```python
from build123d import *

# Parameters (mm, degrees)
RESSALTO_EXTRUS_O1_DEPTH = 50
ESBO_O2_R                = 4
CORTE_EXTRUS_O1_DEPTH    = 24
CORTE_EXTRUS_O2_DEPTH    = 51
FILETE1_R                = 10


with BuildPart() as part:
    # Esboço1 → Ressalto-extrusão1 (new body)
    with BuildSketch(Plane.XY):
        Polygon((87.5, 0), (-87.5, 0), (-87.5, 23), (-20, 23), (-20, 85), (20, 85), (20, 23), (87.5, 23), align=None)
    extrude(amount=RESSALTO_EXTRUS_O1_DEPTH)

    # Esboço2 → Corte-extrusão1 (cut, through all)
    with BuildSketch(Plane(origin=(0, 23, 0), x_dir=(1, 0, 0), z_dir=(0, 1, 0))):
        with Locations((-67.5, -25)):
            Circle(ESBO_O2_R)
        with Locations((67.5, -25)):
            Circle(ESBO_O2_R)
    extrude(amount=-CORTE_EXTRUS_O1_DEPTH, mode=Mode.SUBTRACT)

    # Esboço3 → Corte-extrusão2 (cut, through all)
    with BuildSketch(Plane.XY.offset(50)):
        with BuildLine():
            Line((1, 62.660568708), (1, 116.5))
            Line((1, 116.5), (-1, 116.5))
            Line((-1, 116.5), (-1, 62.660568708))
            ThreePointArc((-1, 62.660568708), (0, 37.3), (1, 62.660568708))
        make_face()
    extrude(amount=-CORTE_EXTRUS_O2_DEPTH, mode=Mode.SUBTRACT)

    # Filete1
    filete1_edges = [part.edges().sort_by_distance(p)[0] for p in [
        (-20, 23, 25),
        (20, 23, 25),
    ]]
    fillet(filete1_edges, radius=FILETE1_R)

    # Esboço5 → Rebaixo para parafuso de máquina com cabeça panela de M61 (revolve, cut)
    with BuildSketch(Plane(origin=(20, 74.5, 25), x_dir=(0, 0, -1), z_dir=(0, 1, 0))):
        Polygon((0, 0), (0, 107.5), (3.3, 107.5), (3.3, 4.6), (6.5, 4.6), (6.5, 0.025), (6.525, 0), align=None)
    revolve(axis=Axis((26.35, 74.5, 25), (-1, 0, 0)), mode=Mode.SUBTRACT)


solid = part.part
```
Input: part model. Units: mm. Frame: model coordinates. A direction names the side the tool comes from. Coordinates: 2 decimals unless noted, no trailing zeros. Loops run counter-clockwise (first coordinate to the right, second up) from the corner with the lowest first, then second, coordinate; pieces in that order, holes last.
Q1. Set-up query: faces 1 (the cylindrical face through (17.72, 80.845, 26.409)), 2 (the flat face through (1, 71, 25)), 3 (the flat face through (-59, 23, 25)), 4 (the flat face through (58, 23, 25)). Return all of +Z, -Z, +X, -X, +Y, -Y with unobstructed straight access to the full face (end or side cutting, diameter ignored); none if empty.
Results are:
face 1: +X
face 2: +Z, -Z, +Y
face 3: +Z, -Z, -X, +Y
face 4: +Z, -Z, +X, +Y
Q2. Line query: line 1 along X through (y, z) = (16.5, 25); line 2 along Z through (x, y) = (-67.5, 12.5); line 3 along X through (y, z) = (81, 37). Output: solid intervals per line, ascending.
Results are:
line 1: x = -87.5 to -71.5, -63.5 to 63.5, 71.5 to 87.5
line 2: z = 0 to 21, 29 to 50
line 3: x = -20 to -1, 1 to 20
Q3. Mould query, pull axis X, two halves, no side actions, for faces 5 (the cylindrical face through (-0.54, 37.31, 25.35)), 6 (the cylindrical face through (71.315, 11.661, 23.799)), 7 (the flat face through (-87.5, 11, 25)), 8 (the cylindrical face through (8.301, 71.717, 23.226)). Classes: +X half, -X half, draft (parallel to the pull), parting line (faces both ways), or undercut.
Results are:
face 5: undercut
face 6: undercut
face 7: -X half
face 8: draft
Q4. Section D-D, the plane z = 5. Return the cut outline in (x, y).
Results are:
outline: (-87.5, 0) - (87.5, 0) - (87.5, 23) - (30, 23) arc R10 cw to (20, 33) - (20, 85) - (1, 85) - (1, 62.66) arc R12.7 cw (long way) to (-1, 62.66) - (-1, 85) - (-20, 85) - (-20, 33) arc R10 cw to (-30, 23) - (-87.5, 23) - close
Q5. Contact query for flat-ended pins moving along their axis: pin 1 (15 mm diameter, centred on y = 55.5, z = 28.5, fed in from -X); pin 2 (10.5 mm diameter, centred on y = 74.5, z = 25, fed in from +X); pin 3 (14.5 mm diameter, centred on y = 71.5, z = 27.5, fed in from +X). Output: stop coordinate, or through.
Results are:
pin 1: stops at x = -20
pin 2: stops at x = 15.4
pin 3: stops at x = 20
Q6. Section A-A, the plane y = 50. Return the cut outline in (x, z), and give its area (3 significant figures).
Results are:
outline: (-20, 0) - (-12.7, 0) - (-12.7, 50) - (-20, 50) - close; (12.7, 0) - (20, 0) - (20, 50) - (12.7, 50) - close
area: 730 mm2
Q7. Section B-B, the plane x = 67.5. Return the cut outline in (y, z).
Results are:
outline: (0, 0) - (23, 0) - (23, 21) - (0, 21) - close; (0, 29) - (23, 29) - (23, 50) - (0, 50) - close
Q8. Section C-C, the plane y = 74.5. Return the cut outline in (x, z) (3 decimals).
Results are:
outline: (-20, 0) - (-1, 0) - (-1, 21.7) - (-20, 21.7) - close; (-20, 28.3) - (-1, 28.3) - (-1, 50) - (-20, 50) - close; (1, 0) - (20, 0) - (20, 18.475) - (19.975, 18.5) - (15.4, 18.5) - (15.4, 21.7) - (1, 21.7) - close; (1, 28.3) - (15.4, 28.3) - (15.4, 31.5) - (19.975, 31.5) - (20, 31.525) - (20, 50) - (1, 50) - close
